Can you work these out from the model? Positions are in its coordinate system, mm. Face numbers are marked on the shaded views. A direction names the side the tool comes from. Give positions to 0.01 mm unless a question says otherwise; leave off trailing zeros. Loops run counter-clockwise (first coordinate to the right, second up) from the corner with the lowest first, then second, coordinate; pieces in that order, holes last. Notation, with made-up numbers: (-29.5, 23) - (-7.5, 23) arc R26 cw to (-7.5, 58) - close; hole circle Ø9 at (-5, 14). An arc over 180 degrees is marked (long way). Answer as a JSON object with one key per item and string values. Group by question number.
Item 1: Which directions (+Z, -Z, +X, -X, +Y, -Y) give clear straight access to the entire face, cutting with the end or side of a thin tool? Please do the marked faces 1 and 2.
Item 2: Thinking about a two-plate mould opening in Y: for the marked faces 3, 4 and 5, which applies, pulls with the +Y half, pulls with the -Y half, needs draft (parallel to the pull), parting line crosses it, or undercut?
Item 3: Please list where these lines run through material, in increasing order: L1, parallel to Y at x = 0, z = 13; L2, parallel to Y at x = 0, z = 2.5; L3, parallel to X at y = 0.75, z = 16.25.
Item 4: Will these pins go through, and if not, where does the flat tip stop? pin 1 (1.5 mm diameter, centred on y = -3.5, z = 6.5, fed in from -X); pin 2 (2 mm diameter, centred on x = 3, z = 6.5, fed in from +Y); pin 3 (1 mm diameter, centred on x = -3, z = 6, fed in from -Y).
Item 5: Suppose I cut it at A-A on x = 0. Write out the boundary of the cut face in (y, z), and give its area (3 significant figures).
Item 6: Suppose I cut it at C-C on z = 9. Write out the boundary of the cut face in (x, y).
Item 7: Suppose I cut it at B-B on y = 0.5. Write out the boundary of the cut face in (x, z), and give its area (3 significant figures).
Item 8: Suppose I cut it at D-D on x = 2.5. Write out the boundary of the cut face in (y, z), and give its area (3 significant figures).
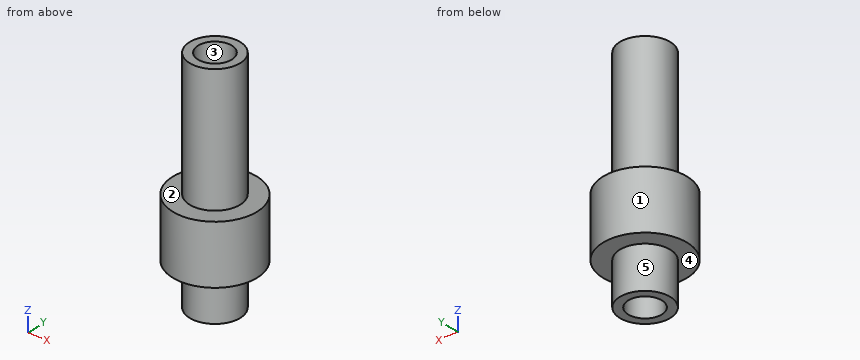
from build123d import *

# Parameters (mm, degrees)
SKETCH_1_R          = 5
EXTRUDE_1_DEPTH     = 7
SKETCH_2_R          = 3
EXTRUDE_2_DEPTH     = 15
EXTRUDE_START       = 5
SKETCH_3_R          = 3
EXTRUDE_3_DEPTH     = 5
SKETCH_4_R          = 2
CUT_EXTRUDE_1_DEPTH = 27


with BuildPart() as part:
    # 스케치1 → 돌출1 (new body)
    with BuildSketch(Plane.XY):
        Circle(SKETCH_1_R)
    extrude(amount=EXTRUDE_1_DEPTH)

    # 스케치2 → 돌출2 (add)
    with BuildSketch(Plane.XY.offset(7)):
        Circle(SKETCH_2_R)
    extrude(amount=EXTRUDE_2_DEPTH)

    # 스케치3 → 돌출3 (add)
    with BuildSketch(Plane(origin=(0, 0, 0), x_dir=(-1, 0, 0), z_dir=(0, 0, -1)).offset(EXTRUDE_START)):
        with Locations(Location((0, 0, 0), (0, 0, 180))):
            Circle(SKETCH_3_R)
    extrude(amount=-EXTRUDE_3_DEPTH)

    # 스케치4 → 컷-돌출1 (cut)
    with BuildSketch(Plane.XY.offset(22)):
        Circle(SKETCH_4_R)
    extrude(amount=-CUT_EXTRUDE_1_DEPTH, mode=Mode.SUBTRACT)


solid = part.part
Worked out:
{
 "1": {"face 1": "+Z, -Z", "face 2": "+Z"},
 "2": {"face 3": "undercut", "face 4": "needs draft", "face 5": "parting line crosses it"},
 "3": {"L1": "y = -3 to -2, 2 to 3", "L2": "y = -5 to -2, 2 to 5", "L3": "x = -2.9 to -1.85, 1.85 to 2.9"},
 "4": {"pin 1": "stops at x = -4.18", "pin 2": "stops at y = 4.58", "pin 3": "stops at y = -4.33"},
 "5": {"outline": "(-5, 0) - (-3, 0) - (-3, -5) - (-2, -5) - (-2, 22) - (-3, 22) - (-3, 7) - (-5, 7) - close; (2, -5) - (3, -5) - (3, 0) - (5, 0) - (5, 7) - (3, 7) - (3, 22) - (2, 22) - close", "area": "82.0 mm2"},
 "6": {"outline": "circle Ø6 at (0, 0); hole circle Ø4 at (0, 0)"},
 "7": {"outline": "(-4.97, 0) - (-2.96, 0) - (-2.96, -5) - (-1.94, -5) - (-1.94, 22) - (-2.96, 22) - (-2.96, 7) - (-4.97, 7) - close; (1.94, -5) - (2.96, -5) - (2.96, 0) - (4.97, 0) - (4.97, 7) - (2.96, 7) - (2.96, 22) - (1.94, 22) - close", "area": "83.4 mm2"},
 "8": {"outline": "(-4.33, 0) - (-1.66, 0) - (-1.66, -5) - (1.66, -5) - (1.66, 0) - (4.33, 0) - (4.33, 7) - (1.66, 7) - (1.66, 22) - (-1.66, 22) - (-1.66, 7) - (-4.33, 7) - close", "area": "127 mm2"}
}
